```python
from build123d import *

# Parameters (mm, degrees)
SKETCH1_W                   = 228.6
SKETCH1_H                   = 72.39
BOSS_EXTRUDE1_DEPTH         = 4.7625
SKETCH2_W                   = 215.9
SKETCH2_H                   = 64.77
SKETCH2_W_2                 = 207.772
SKETCH2_H_2                 = 56.642
CUT_EXTRUDE1_DEPTH          = 2.794
FILLET1_R                   = 9.525
FILLET2_R                   = 6.35
F_19_0_166_DIAMETER_HOLE1_D = 4.2164
LPATTERN1_COUNT             = 2
LPATTERN1_PITCH             = 219.075
LPATTERN1_COUNT_DIR2        = 2
LPATTERN1_PITCH_DIR2        = 63.5


with BuildPart() as part:
    # Sketch1 → Boss-Extrude1 (new body)
    with BuildSketch(Plane(origin=(0, 0, 0), x_dir=(1, 0, 0), z_dir=(0, 1, 0))):
        with Locations((114.3, 36.195)):
            Rectangle(SKETCH1_W, SKETCH1_H)
    extrude(amount=BOSS_EXTRUDE1_DEPTH)

    # Sketch2 → Cut-Extrude1 (cut)
    with BuildSketch(Plane(origin=(0, 4.7625, 0), x_dir=(1, 0, 0), z_dir=(0, 1, 0))):
        with Locations((114.3, 36.195)):
            Rectangle(SKETCH2_W, SKETCH2_H)
        with Locations((114.3, 36.195)):
            Rectangle(SKETCH2_W_2, SKETCH2_H_2, mode=Mode.SUBTRACT)
    extrude(amount=-CUT_EXTRUDE1_DEPTH, mode=Mode.SUBTRACT)

    # Fillet1
    fillet1_edges = [part.edges().sort_by_distance(p)[0] for p in [
        (6.35, 3.3655, -3.81),
        (6.35, 3.3655, -68.58),
        (222.25, 3.3655, -68.58),
        (222.25, 3.3655, -3.81),
    ]]
    fillet(fillet1_edges, radius=FILLET1_R)

    # Fillet2
    fillet2_edges = [part.edges().sort_by_distance(p)[0] for p in [
        (10.414, 3.3655, -64.516),
        (218.186, 3.3655, -64.516),
        (218.186, 3.3655, -7.874),
        (10.414, 3.3655, -7.874),
    ]]
    fillet(fillet2_edges, radius=FILLET2_R)

    # #19 (0.166) Diameter Hole1 (through all)
    with Locations(Plane(origin=(0, 4.7625, 0), x_dir=(1, 0, 0), z_dir=(0, 1, 0))):
        with Locations((4.7625, 4.445)):
            f_19_0_166_diameter_hole1 = Hole(F_19_0_166_DIAMETER_HOLE1_D / 2)

    # LPattern1: 19 _0.166_ Diameter Hole1 2 × 2
    with Locations(*[(i * LPATTERN1_PITCH, 0, -j * LPATTERN1_PITCH_DIR2) for i in range(LPATTERN1_COUNT) for j in range(LPATTERN1_COUNT_DIR2) if (i, j) != (0, 0)]):
        add(f_19_0_166_diameter_hole1, mode=Mode.SUBTRACT)


solid = part.part
```
For this review, take the finished solid that the model builds, in its own axes (mm). A direction names the side the tool comes from. Give positions to 0.01 mm unless a question says otherwise; leave off trailing zeros. Write each loop counter-clockwise with the first axis right and the second up, starting at its lowest first coordinate (ties: lowest second). Pieces come first, ordered by that corner, then holes.
Item 1: The part is to be moulded in two halves that separate along X. For faces 1 (the face through (113, 2, -72.39)), 2 (the face through (0, 2, -36)), 3 (the face through (6.87, 2.35, -4.54)), say which applies: +X half, -X half, draft (parallel to the pull), parting line (faces both ways), or undercut.
Item 2: Machinability: for faces 4 (the face through (221.89, 2.35, -3.64)), 5 (the face through (12.324, 3.346, -62.705)), which of the approach directions +Z, -Z, +X, -X, +Y, -Y give a long, thin tool a straight path to every point of the face, cutting with its end or side? Answer none if there is none.
Item 3: Take a section at A-A (y = 3.4). Give the number of separate pieces and of enclosed holes in the cut face, and give its area (3 significant figures).
Item 4: Insertion check: P1, Ø2, axis at y = 3, z = -27, coming from the -X side. The pin has a flat end and moves straight along its axis. Give the tip position at first contact, or say it passes through.
Item 5: Take a section at B-B (x = 120.5). Give the boundary of the cut face in (y, z), and give its area (3 significant figures).
Item 6: Take a section at C-C (z = -34). Give the boundary of the cut face in (x, y), and give its area (3 significant figures).
Item 7: Wall thickness on probe 1 along Z at (x, y) = (45, 3.35); probe 2 along X at (y, z) = (3.35, -47.5); probe 3 along X at (y, z) = (2.3, -8.5): over which ranges is each line inside the solid? List them lowest first.
Established:
1. face 1: draft
1. face 2: -X half
1. face 3: undercut
2. face 4: +Y, -Y
2. face 5: +Y
3. separate pieces: 2
3. enclosed holes: 5
3. area: 14,300 mm2
4. P1: stops at x = 0
5. outline: (0, -72.39) - (4.76, -72.39) - (4.76, -68.58) - (1.97, -68.58) - (1.97, -64.52) - (4.76, -64.52) - (4.76, -7.87) - (1.97, -7.87) - (1.97, -3.81) - (4.76, -3.81) - (4.76, 0) - (0, 0) - close
5. area: 322 mm2
6. outline: (0, 0) - (228.6, 0) - (228.6, 4.76) - (222.25, 4.76) - (222.25, 1.97) - (218.19, 1.97) - (218.19, 4.76) - (10.41, 4.76) - (10.41, 1.97) - (6.35, 1.97) - (6.35, 4.76) - (0, 4.76) - close
6. area: 1,070 mm2
7. probe 1: z = -72.39 to -68.58, -64.52 to -7.87, -3.81 to 0
7. probe 2: x = 0 to 6.35, 10.41 to 218.19, 222.25 to 228.6
7. probe 3: x = 0 to 7.67, 14.01 to 214.59, 220.93 to 228.6
